Read the model definition and answer for the solid it produces. Units are mm, in the model's axes. A direction names the side the tool comes from. Coordinates: 2 decimals unless noted, no trailing zeros. Order: outer loops, then holes, each group sorted by start corner. A loop starts at its lowest first (then second) coordinate and runs counter-clockwise, first axis right, second up. Notation, with made-up numbers: (87.5, 49.5) -> (91.5, 49.5) arc R15 ccw to (91.5, 62.5) -> close; hole circle Ø5 at (79, -18). An arc over 180 degrees is marked (long way). Answer in a Markdown table with one row per item.
from build123d import *

# Parameters (mm, degrees)
F0_R     = 50.8
F0_R_2   = 19.05
F1_DEPTH = 101.6
F0_R_3   = 76.2
F2_DEPTH = 6.35
F7_R     = 3.175
F8_DEPTH = 25.4


with BuildPart() as f1:
    # F0 (on Front) → F1 (new body)
    with BuildSketch(Plane.XZ):
        Circle(F0_R)
        Circle(F0_R_2, mode=Mode.SUBTRACT)
    extrude(amount=F1_DEPTH)

    # F0 (on Front) → F2 (join)
    with BuildSketch(Plane.XZ):
        Circle(F0_R_3)
        Circle(F0_R, mode=Mode.SUBTRACT)
    extrude(amount=F2_DEPTH)

    # F3 (on Right) → F4 (revolve, cut)
    with BuildSketch(Plane.YZ):
        Polygon((-109.346762, 21.367406), (-6.33552, 50.977927), (-107.67857, 54.314323), align=None)
    revolve(axis=Axis((0, -101.6, 0), (0, -1, 0)), mode=Mode.SUBTRACT)

    # F5 (on Top) → F6 (revolve, cut)
    with BuildSketch(Plane.XY):
        Polygon((-55.385999, -52.059986), (-25.6285, -95.704317), (-25.6285, -88.51292), (-21.660833, -83.305359), (-32.501825, -75.045552), (-25.6285, -66.024315), (-37.851702, -56.711396), (-31.398905, -48.242103), (-43.97326, -38.661638), (-37.03554, -25.526214), (-49.323034, -19.036344), (-52.410249, -6.6798), align=None)
    revolve(axis=Axis((0, -101.6, 0), (0, 1, 0)), mode=Mode.SUBTRACT)

    # F7 (on face) → F8 (cut)
    with BuildSketch(Plane.XZ.offset(6.35)):
        with Locations((0, 64.114898)):
            Circle(F7_R)
        with Locations((45.336079, 45.336079)):
            Circle(F7_R)
        with Locations((-45.336079, 45.336079)):
            Circle(F7_R)
        with Locations((-64.114898, 0)):
            Circle(F7_R)
        with Locations((64.114898, 0)):
            Circle(F7_R)
        with Locations((45.336079, -45.336079)):
            Circle(F7_R)
        with Locations((0, -64.114898)):
            Circle(F7_R)
        with Locations((-45.336079, -45.336079)):
            Circle(F7_R)
    extrude(amount=-F8_DEPTH, mode=Mode.SUBTRACT)


solid = f1.part
Q1. Given pin 1 (7.5 mm diameter, centred on x = 45.34, z = -45.34, fed in from +Y); pin 2 (10 mm diameter, centred on x = -64.11, z = 0, fed in from -Y); pin 3 (6 mm diameter, centred on x = 29, y = -13, fed in from -Z); pin 4 (12 mm diameter, centred on x = -18, y = -80, fed in from +Z), each flat-ended and moving along its own axis, determine where each tip first touches the part or whether it passes through.
Outcome:
| item | result |
|---|---|
| pin 1 | y = 0 |
| pin 2 | y = -6.35 |
| pin 3 | z = -41.86 |
| pin 4 | z = 27.86 |
Q2. The part is cut by section C-C (y = -9.5). Write down the section's boundary in (x, z).
Outcome:
| item | result |
|---|---|
| outline | circle Ø100.14 at (0, 0); hole circle Ø38.1 at (0, 0) |
Q3. Consider line 1 (Z direction, x = 0, y = -5); line 2 (Y direction, x = 14, z = 64); line 3 (X direction, y = -74.5, z = -4.5). Determine where each line is inside the solid, lowest interval first.
Outcome:
| item | result |
|---|---|
| line 1 | -76.2 to -67.29, -60.94 to -19.05, 19.05 to 60.94, 67.29 to 76.2 |
| line 2 | -6.35 to 0 |
| line 3 | -31.06 to -18.51, 18.51 to 31.06 |
Q4. For a pull along X with two mould halves and no side action, classify faces 4 (the face through (8.086, -26.028, -36.413)), 5 (the face through (1.71, -3.22, 66.79)), 6 (the face through (16, 0, -16)) as pulls with the +X half, pulls with the -X half, needs draft (parallel to the pull), parting line crosses it, or undercut.
Outcome:
| item | result |
|---|---|
| face 4 | parting line crosses it |
| face 5 | undercut |
| face 6 | needs draft |
Q5. The part is cut by section B-B (z = 0). Give the number of separate pieces and of enclosed holes in the cut face, then the cut area to 3 significant figures.
Outcome:
| item | result |
|---|---|
| separate pieces | 4 |
| enclosed holes | 0 |
| area | 3,640 mm² |
Q6. For faces 1 (the face through (-16, -101.6, 11)), 2 (the face through (5.698, -65.524, -25.66)), 3 (the face through (5.56, -91.48, -25.02)), determine the directions among +Z, -Z, +X, -X, +Y, -Y from which every point of the face is accessible in a straight line to the end or side of a thin tool.
Outcome:
| item | result |
|---|---|
| face 1 | +Z, -Z, +X, -X, -Y |
| face 2 | none |
| face 3 | -Y |
Q7. The part is cut by section A-A (x = -65). Write down the section's boundary in (y, z).
Outcome:
| item | result |
|---|---|
| outline | (-6.35, -39.77) -> (0, -39.77) -> (0, -3.05) -> (-6.35, -3.05) -> close; (-6.35, 3.05) -> (0, 3.05) -> (0, 39.77) -> (-6.35, 39.77) -> close |
